Part model, mm, in its own coordinate system. A direction names the side the tool comes from. Coordinates: 2 decimals unless noted, no trailing zeros. Write each loop counter-clockwise with the first axis right and the second up, starting at its lowest first coordinate (ties: lowest second). Pieces come first, ordered by that corner, then holes. Notation, with made-up numbers: (-11.5, -40) -> (-3.5, -40) arc R24 cw to (-3.5, -14) -> close; hole circle Ø3 at (80.25, 33.25). An arc over 180 degrees is marked (long way). Write item = value, one per line. Start each with the question number.
Q1. Tool access for faces 1 (the flat face through (0, -6.35, 157)), 2 (the flat face through (0, 4.762, 157)): list every direction of +Z, -Z, +X, -X, +Y, -Y with a clear straight run to the whole face (end or side of a thin tool).
Q2. Pin check, flat tips, straight feed: P1, Ø7.5, axis at y = 0, z = 6.35, coming from the +X side; P2, Ø4, axis at y = 0, z = 6.35, coming from the -X side. Stop position of each tip, or through.
Q3. Band-saw the part on A-A, the plane x = -2.25. List the corners of the cut face in (y, z).
Q4. Pull direction Z, two halves, no side cores. Call faces 3 (the flat face through (6, 0, 0)), 4 (the cylindrical face through (-5.545, 1.707, 9.027)), 5 (the cylindrical face through (-5.545, 1.707, 313.827)), 6 (the flat face through (6.35, 0, 157)): released by +Z, released by -Z, zero draft, split by the parting line, or undercut.
Q5. Probe line 1 (Z direction, x = 5.6, y = 0) (3 decimals); line 2 (Y direction, x = -4.5, z = 71). List the from-to ranges inside material, lowest first.
Q6. Band-saw the part on C-C, the plane y = 0. Give the number of separate pieces and of enclosed holes in the cut face, plus the area to 3 significant figures.
Q7. Band-saw the part on B-B, the plane z = 126. List the corners of the cut face in (x, y), plus the area to 3 significant figures.
from build123d import *

# Parameters (mm, degrees)
F1_DEPTH = 317.5
F2_R     = 3.175
F3_DEPTH = 12.701


with BuildPart() as f1:
    # F0 (on Top) → F1 (new body)
    with BuildSketch(Plane.XY):
        Polygon((0, 4.7625), (4.7625, 4.7625), (4.7625, 0), (6.35, 0), (6.35, 6.35), (0, 6.35), align=None)
        Polygon((-4.7625, 4.7625), (0, 4.7625), (0, 6.35), (-6.35, 6.35), (-6.35, -6.35), (6.35, -6.35), (6.35, 0), (4.7625, 0), (4.7625, -4.7625), (-4.7625, -4.7625), align=None)
    extrude(amount=F1_DEPTH)

    # F2 (on face) → F3 (cut, through all)
    with BuildSketch(Plane.YZ.offset(6.35)):
        with Locations((0, 6.35)):
            Circle(F2_R)
        with Locations((0, 311.15)):
            Circle(F2_R)
    extrude(amount=-F3_DEPTH, mode=Mode.SUBTRACT)


solid = f1.part
Ans:
q1.face_1 = +Z, -Z, +X, -X, -Y
q1.face_2 = +Z, -Z
q2.P1 = 6.35
q2.P2 = through
q3.outline = (-6.35, 0) -> (-4.76, 0) -> (-4.76, 317.5) -> (-6.35, 317.5) -> close; (4.76, 0) -> (6.35, 0) -> (6.35, 317.5) -> (4.76, 317.5) -> close
q4.face_3 = released by -Z
q4.face_4 = undercut
q4.face_5 = undercut
q4.face_6 = zero draft
q5.line_1 = 0 to 3.175, 9.525 to 307.975, 314.325 to 317.5
q5.line_2 = -6.35 to -4.76, 4.76 to 6.35
q6.separate_pieces = 6
q6.enclosed_holes = 0
q6.area = 968 mm2
q7.outline = (-6.35, -6.35) -> (6.35, -6.35) -> (6.35, 6.35) -> (-6.35, 6.35) -> close; hole (-4.76, -4.76) -> (4.76, -4.76) -> (4.76, 4.76) -> (-4.76, 4.76) -> close
q7.area = 70.6 mm2
